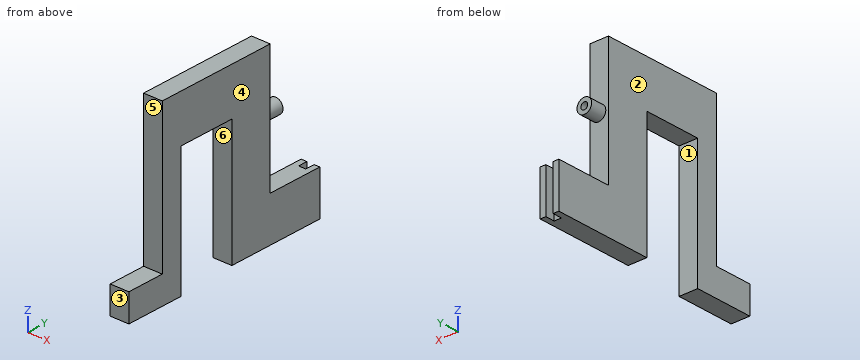
```python
from build123d import *

# Parameters (mm, degrees)
F1_DEPTH = 20
F2_W     = 7.7429511584
F2_H     = 47.2369704668
F3_DEPTH = 10
F4_R     = 7.8502979612
F4_R_2   = 3.6441715019
F5_DEPTH = 17


with BuildPart() as f1:
    # F0 (on Right) → F1 (new body)
    with BuildSketch(Plane.YZ):
        Polygon((-41.4293780923, -31.1796526851), (-81.5630704165, -31.1796526851), (-81.5630704165, -60.4142908512), (-18.9877006452, -60.4142908512), (-18.9877006452, 76.117331113), (42.1743764823, 76.117331113), (42.1743764823, -56.8378705173), (147.8243358508, -56.8378705173), (147.8243358508, -9.6009000506), (88.1971307173, -9.6009000506), (88.1971307173, 125.9854882991), (-41.4293780923, 125.9854882991), align=None)
    extrude(amount=F1_DEPTH)

    # F2 (on face) → F3 (cut)
    with BuildSketch(Plane(origin=(0, 147.8243358508, 0), x_dir=(-1, 0, 0), z_dir=(0, 1, 0))):
        with Locations((-10.0561461877, -33.2193852839)):
            Rectangle(F2_W, F2_H)
    extrude(amount=-F3_DEPTH, mode=Mode.SUBTRACT)

    # F4 (on face) → F5 (join)
    with BuildSketch(Plane(origin=(0, 88.1971307173, 0), x_dir=(-1, 0, 0), z_dir=(0, 1, 0))):
        with Locations((-10.7497964054, 59.6960298717)):
            Circle(F4_R)
        with Locations((-10.7497964054, 59.6960298717)):
            Circle(F4_R_2, mode=Mode.SUBTRACT)
    extrude(amount=F5_DEPTH)


solid = f1.part
```
Check sheet for the modelled part. Datum: model origin and axes. Units: mm. Face numbers are marked on the shaded views. A direction names the side the tool comes from. Coordinates: 2 decimals unless noted, no trailing zeros. Write each loop counter-clockwise with the first axis right and the second up, starting at its lowest first coordinate (ties: lowest second). Pieces come first, ordered by that corner, then holes. Notation, with made-up numbers: (69.5, 72) -> (111.5, 72) arc R38 ccw to (111.5, 111) -> close; hole circle Ø1 at (-21, -32.5). An arc over 180 degrees is marked (long way). Use a Markdown table: item, result.
1. Release check for a two-part mould opening along Y. For the marked faces 1, 2 and 3 record: pulls with the +Y half, pulls with the -Y half, needs draft (parallel to the pull), parting line crosses it, or undercut.
Reported:
| item | result |
|---|---|
| face 1 | undercut |
| face 2 | needs draft |
| face 3 | pulls with the -Y half |
2. Sectioned sample at B-B (z = -48). Enter the section's corners in (x, y).
Reported:
| item | result |
|---|---|
| outline | (0, -81.56) -> (20, -81.56) -> (20, -18.99) -> (0, -18.99) -> close; (0, 42.17) -> (20, 42.17) -> (20, 147.82) -> (13.93, 147.82) -> (13.93, 137.82) -> (6.18, 137.82) -> (6.18, 147.82) -> (0, 147.82) -> close |
3. Sectioned sample at C-C (y = 128). Enter the section's corners in (x, z), plus the area to 3 significant figures.
Reported:
| item | result |
|---|---|
| outline | (0, -56.84) -> (20, -56.84) -> (20, -9.6) -> (0, -9.6) -> close |
| area | 945 mm2 |
4. Scan lines: line 1 along Y through (x, z) = (11.25, -45.5); line 2 along Y through (x, z) = (5, 29); line 3 along Z through (x, y) = (11, 103.5). Record each from-to range of solid material in increasing order.
Reported:
| item | result |
|---|---|
| line 1 | y = -81.56 to -18.99, 42.17 to 137.82 |
| line 2 | y = -41.43 to -18.99, 42.17 to 88.2 |
| line 3 | z = -56.84 to -9.6, 51.85 to 56.06, 63.33 to 67.54 |
5. Sectioned sample at D-D (z = 89). Enter the section's corners in (x, y).
Reported:
| item | result |
|---|---|
| outline | (0, -41.43) -> (20, -41.43) -> (20, 88.2) -> (0, 88.2) -> close |
6. Sectioned sample at A-A (z = 33.5). Enter the section's corners in (x, y).
Reported:
| item | result |
|---|---|
| outline | (0, -41.43) -> (20, -41.43) -> (20, -18.99) -> (0, -18.99) -> close; (0, 42.17) -> (20, 42.17) -> (20, 88.2) -> (0, 88.2) -> close |
7. Go/stop test with flat-tipped pins: pin 1 Ø11.5 at (x, z) = (10.75, 59.7) entering from -Y; pin 2 Ø10 at (x, y) = (14, 111.5) entering from +Z; pin 3 Ø6 at (x, z) = (12, 37) entering from +Y; pin 4 Ø1.5 at (y, z) = (-43, -23.5) entering from +X. Record where each tip stops, or that it passes through.
Reported:
| item | result |
|---|---|
| pin 1 | stops at y = -41.43 |
| pin 2 | stops at z = -9.6 |
| pin 3 | stops at y = 88.2 |
| pin 4 | passes through |
8. Tool access check on the marked faces 4, 5 and 6. Record the directions out of +Z, -Z, +X, -X, +Y, -Y that give a thin tool (end or side, any length) a straight path to the whole face; none if there is none.
Reported:
| item | result |
|---|---|
| face 4 | +Z, -Z, +X, +Y, -Y |
| face 5 | +Z, +X, -X, -Y |
| face 6 | -Z, +X, -X |
